Autodesk Inventor part; units mm, degrees
ref_plane "Work Plane1" through (0, 0, 13) normal (0, 0, -1) x (-1, 0, 0)
ref_plane "YZ Plane" through (0, 0, 0) normal (1, 0, 0) x (0, 1, 0)
ref_plane "XZ Plane" through (0, 0, 0) normal (0, 1, 0) x (-1, 0, 0)
sketch "Sketch1" plane through (0, 0, 0) normal (0, 0, 1) x (1, 0, 0)
  line L0 (-9.5, -7.5) -> (9.5, -7.5)
  line L1 (9.5, -7.5) -> (9.5, 7.5)
  line L2 (9.5, 7.5) -> (-9.5, 7.5)
  line L3 (-9.5, 7.5) -> (-9.5, -7.5)
  line L4 (-9.5, -7.5) -> (9.5, 7.5) construction
  line L5 (9.5, -7.5) -> (-9.5, 7.5) construction
  point P0 (0, 0)
  dimension "d0" = 19
  dimension "d1" = 15
extrude "Extrusion1" add sketch "Sketch1" along normal blind 1.6
sketch "Sketch2" plane through (0, 0, 0) normal (0, 0, -1) x (-1, 0, 0)
  line L0 (0, -10.5) -> (0, 10.5)
  line L1 (-8.5, -6.5) -> (8.5, -6.5)
  line L2 (8.5, -6.5) -> (8.5, -1.5)
  line L3 (8.5, -1.5) -> (-8.5, -1.5)
  line L4 (-8.5, -1.5) -> (-8.5, -6.5)
  line L5 (-8.5, -6.5) -> (8.5, -1.5) construction
  line L6 (8.5, -6.5) -> (-8.5, -1.5) construction
  line L7 (9.5, -7.5) -> (-9.5, -7.5)
  point P0 (0, 0)
  point P1 (0, -4)
  dimension "d4" = 5
  dimension "d5" = 1
  dimension "d6" = 17
extrude "Extrusion2" add sketch "Sketch2" along normal blind 2
sketch "Sketch3" plane through (0, 0, 1.6) normal (0, 0, 1) x (1, 0, 0)
  line L0 (0, -10.5) -> (0, 10.5)
  line L1 (-7, 1.5) -> (7, 1.5)
  line L2 (7, 1.5) -> (7, 5.5)
  line L3 (7, 5.5) -> (-7, 5.5)
  line L4 (-7, 5.5) -> (-7, 1.5)
  line L5 (-7, 1.5) -> (7, 5.5) construction
  line L6 (7, 1.5) -> (-7, 5.5) construction
  line L7 (9.5, 7.5) -> (-9.5, 7.5)
  point P0 (0, 0)
  point P1 (0, 3.5)
  dimension "d9" = 14
  dimension "d10" = 4
  dimension "d11" = 2
ref_plane "Work Plane1" through (0, 0, 13) normal (0, 0, -1) x (-1, 0, 0)
extrude "Extrusion3" add sketch "Sketch3" along normal up to surface (11.4 mm away)
sketch "Sketch4" plane through (-7, 1.5, 13) normal (0, 0, 1) x (1, 0, 0)
  line L0 (0, 4) -> (0, 0)
  line L1 (0, 0) -> (14, 0)
  line L2 (14, 0) -> (14, 4)
  line L3 (14, 4) -> (0, 4)
  line L4 (0, 1.492) -> (1.5696, 1.492)
  line L5 (1.5696, 1.492) -> (2.677, 0)
  line L6 (7, -12) -> (7, 9) construction
  line L7 (14, 1.492) -> (12.4304, 1.492)
  line L8 (12.4304, 1.492) -> (11.323, 0)
  point P0 (7, -1.5)
extrude "Extrusion4" cut sketch "Sketch4" against normal blind 8.25 contours L4 L5 L1 L0 | L2 L1 L8 L7
fillet "Fillet1" radius 0.5 10 edges at (7, 5.5, 7.3) (-7, 5.5, 7.3) (7, 2.992, 8.875) (4.323, 1.5, 8.875) (-7, 2.992, 8.875) (-4.323, 1.5, 8.875) (-5.4304, 2.992, 8.875) (5.4304, 2.992, 8.875) (7, 1.5, 3.175) (-7, 1.5, 3.175)
properties part number "Adafruit_L_Bend_HDMI_Plug_Adapter_3550"
CAD build for the part. Positions are in the model's coordinates, mm. A direction names the side the tool comes from. Give positions to 0.01 mm unless a question says otherwise; leave off trailing zeros. Loops run counter-clockwise (first coordinate to the right, second up) from the corner with the lowest first, then second, coordinate; pieces in that order, holes last. Notation, with made-up numbers: (56, 51.5) -> (78, 51.5) arc R19 cw to (78, 57.5) -> close; hole circle Ø10 at (65.25, 23.5). An arc over 180 degrees is marked (long way). Use a Markdown table: item, result.
1. Slice it at A-A (z = 2). List the corners of the cut face in (x, y).
Check result:
| item | result |
|---|---|
| outline | (-7, 2) arc R0.5 ccw to (-6.5, 1.5) -> (6.5, 1.5) arc R0.5 ccw to (7, 2) -> (7, 5) arc R0.5 ccw to (6.5, 5.5) -> (-6.5, 5.5) arc R0.5 ccw to (-7, 5) -> close |
2. Slice it at D-D (z = 11.5). List the corners of the cut face in (x, y), plus the area to 3 significant figures.
Check result:
| item | result |
|---|---|
| outline | (-7, 3.49) arc R0.5 ccw to (-6.5, 2.99) -> (-5.68, 2.99) arc R0.5 cw to (-5.28, 2.79) -> (-4.47, 1.7) arc R0.5 ccw to (-4.07, 1.5) -> (4.07, 1.5) arc R0.5 ccw to (4.47, 1.7) -> (5.28, 2.79) arc R0.5 cw to (5.68, 2.99) -> (6.5, 2.99) arc R0.5 ccw to (7, 3.49) -> (7, 5) arc R0.5 ccw to (6.5, 5.5) -> (-6.5, 5.5) arc R0.5 ccw to (-7, 5) -> close |
| area | 49.4 mm^2 |
3. Which spindle directions (+Z, -Z, +X, -X, +Y, -Y) get a long thin tool onto all of the face, cutting with end or side? Do faces 1 (the flat face through (8.5, -4, -1)), 2 (the flat face through (0, 1.5, 6)), 3 (the flat face through (6, 2.992, 9)), 4 (the flat face through (-4.88, 2.25, 8.93)). Say none if no direction does.
Check result:
| item | result |
|---|---|
| face 1 | -Z, +X, +Y, -Y |
| face 2 | +Z, +X, -X, -Y |
| face 3 | +Z, +X, -Y |
| face 4 | +Z, -X, -Y |
4. Flat gauge pins, fed straight in: pin 1 (1.5 mm diameter, centred on y = 5, z = 6.5, fed in from -X); pin 2 (2 mm diameter, centred on y = 1, z = 3.5, fed in from +X); pin 3 (4.5 mm diameter, centred on x = -4, y = -2, fed in from +Z). Where does each tip first touch, or does it go through?
Check result:
| item | result |
|---|---|
| pin 1 | stops at x = -7 |
| pin 2 | stops at x = 7 |
| pin 3 | stops at z = 1.6 |
5. Wall check: L1, parallel to Y at x = -0.5, z = -0.75; L2, parallel to Y at x = 1.5, z = 12.5; L3, parallel to Z at x = 2, y = -2.25. Give the ranges that are in metal, low to high. Write a range as [from, to].
Check result:
| item | result |
|---|---|
| L1 | y = [-6.5, -1.5] |
| L2 | y = [1.5, 5.5] |
| L3 | z = [-2, 1.6] |
6. Slice it at B-B (x = -1.5). List the corners of the cut face in (y, z).
Check result:
| item | result |
|---|---|
| outline | (-7.5, 0) -> (-6.5, 0) -> (-6.5, -2) -> (-1.5, -2) -> (-1.5, 0) -> (7.5, 0) -> (7.5, 1.6) -> (5.5, 1.6) -> (5.5, 13) -> (1.5, 13) -> (1.5, 1.6) -> (-7.5, 1.6) -> close |
7. Slice it at C-C (y = -6). List the corners of the cut face in (x, z).
Check result:
| item | result |
|---|---|
| outline | (-9.5, 0) -> (-8.5, 0) -> (-8.5, -2) -> (8.5, -2) -> (8.5, 0) -> (9.5, 0) -> (9.5, 1.6) -> (-9.5, 1.6) -> close |
